The listing builds one solid part. Answer for the finished solid, in the listing's coordinates (mm). Face numbers are marked on the shaded views. A direction names the side the tool comes from. Round coordinates to 2 decimals unless told otherwise and drop trailing zeros. Order: outer loops, then holes, each group sorted by start corner. A loop starts at its lowest first (then second) coordinate and runs counter-clockwise, first axis right, second up. Notation, with made-up numbers: (82, -34.5) - (99, -34.5) arc R14 cw to (99, -12.5) - close; hole circle Ø10 at (19, 67). An arc over 180 degrees is marked (long way). One line per item, written item: value. Start each with the question number.
1. Flat-ended cylindrical pins translate along their axes: P1, Ø3, axis at x = 7.91, z = 6.66, coming from the -Y side (3 decimals); P2, Ø14.5, axis at x = 5.5, y = 63.5, coming from the +Z side; P3, Ø4.5, axis at x = -7.09, z = 6.66, coming from the +Y side; P4, Ø2.5, axis at x = -6, z = 6, coming from the -Y side. Find the tip coordinate at first contact, or state that the pin passes through.
2. A tool of negligible diameter and unlimited length cuts with its end or side. For the marked faces 1 and 2, from which of +Z, -Z, +X, -X, +Y, -Y can it reach the whole face along a straight path? Write none if from no direction.
3. Section C-C, the plane x = 6.5 is taken. Give the vertices of the cut face in (y, z).
4. Straight lines are drawn through the part: line 1 (X direction, y = 50, z = 0.75); line 2 (Y direction, x = 10.5, z = 1); line 3 (Z direction, x = 3, y = 45). For each, find the intervals that lie inside material, in ascending order.
5. Section B-B, the plane z = 1 is taken. Give the vertices of the cut face in (x, y), then the cut area to 3 significant figures.
6. Section D-D, the plane z = 5.5 is taken. Give the vertices of the cut face in (x, y).
7. Section A-A, the plane y = 48 is taken. Give the vertices of the cut face in (x, z), then the cut area to 3 significant figures.
from build123d import *

# Parameters (mm, degrees)
SKETCH1_W           = 28.9
SKETCH1_H           = 33
SKETCH1_R           = 2.7
BOSS_EXTRUDE1_DEPTH = 2
FILLET1_R           = 5
SKETCH3_W           = 28.9
SKETCH3_H           = 2
BOSS_EXTRUDE3_DEPTH = 8
SKETCH5_R           = 2
CUT_EXTRUDE2_DEPTH  = 10


with BuildPart() as part:
    # Sketch1 → Boss-Extrude1 (new body)
    with BuildSketch(Plane.XY):
        with Locations((0.904740234, 58.092544957)):
            Rectangle(SKETCH1_W, SKETCH1_H)
        with Locations((-8.545259766, 49.592544957)):
            Circle(SKETCH1_R, mode=Mode.SUBTRACT)
        with Locations((10.354740234, 49.592544957)):
            Circle(SKETCH1_R, mode=Mode.SUBTRACT)
    extrude(amount=BOSS_EXTRUDE1_DEPTH)

    # Fillet1
    fillet1_edges = [part.edges().sort_by_distance(p)[0] for p in [
        (15.354740234, 41.592544957, 1),
        (-13.545259766, 41.592544957, 1),
    ]]
    fillet(fillet1_edges, radius=FILLET1_R)

    # Sketch3 → Boss-Extrude3 (add)
    with BuildSketch(Plane.XY.offset(2)):
        with Locations((0.904740234, 73.592544957)):
            Rectangle(SKETCH3_W, SKETCH3_H)
    extrude(amount=BOSS_EXTRUDE3_DEPTH)

    # Sketch5 → Cut-Extrude2 (cut)
    with BuildSketch(Plane(origin=(0, 74.592544957, 0), x_dir=(1, 0, 0), z_dir=(0, 1, 0))):
        with Locations((-7.091615714, -6.658195947)):
            Circle(SKETCH5_R)
        with Locations((7.908384286, -6.658195947)):
            Circle(SKETCH5_R)
    extrude(amount=-CUT_EXTRUDE2_DEPTH, mode=Mode.SUBTRACT)


solid = part.part
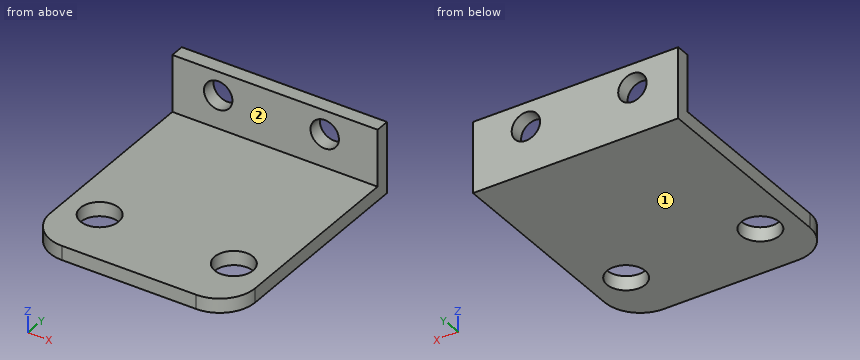
Answer list:
1. P1: passes through
1. P2: stops at z = 2
1. P3: stops at y = 74.59
1. P4: stops at y = 72.59
2. face 1: -Z, +X, -X, +Y, -Y
2. face 2: +Z, +X, -X, -Y
3. outline: (41.59, 0) - (74.59, 0) - (74.59, 5.24) - (72.59, 5.24) - (72.59, 2) - (41.59, 2) - close; (72.59, 8.08) - (74.59, 8.08) - (74.59, 10) - (72.59, 10) - close
4. line 1: x = -13.55 to -11.21, -5.88 to 7.69, 13.02 to 15.35
4. line 2: y = 41.59 to 46.9, 52.29 to 74.59
4. line 3: z = 0 to 2
5. outline: (-13.55, 46.59) arc R5 ccw to (-8.55, 41.59) - (10.35, 41.59) arc R5 ccw to (15.35, 46.59) - (15.35, 74.59) - (-13.55, 74.59) - close; hole circle Ø5.4 at (-8.55, 49.59); hole circle Ø5.4 at (10.35, 49.59)
5. area: 897 mm²
6. outline: (-13.55, 72.59) - (-8.72, 72.59) - (-8.72, 74.59) - (-13.55, 74.59) - close; (-5.46, 72.59) - (6.28, 72.59) - (6.28, 74.59) - (-5.46, 74.59) - close; (9.54, 72.59) - (15.35, 72.59) - (15.35, 74.59) - (9.54, 74.59) - close
7. outline: (-13.55, 0) - (-10.73, 0) - (-10.73, 2) - (-13.55, 2) - close; (-6.36, 0) - (8.17, 0) - (8.17, 2) - (-6.36, 2) - close; (12.54, 0) - (15.35, 0) - (15.35, 2) - (12.54, 2) - close
7. area: 40.4 mm²
